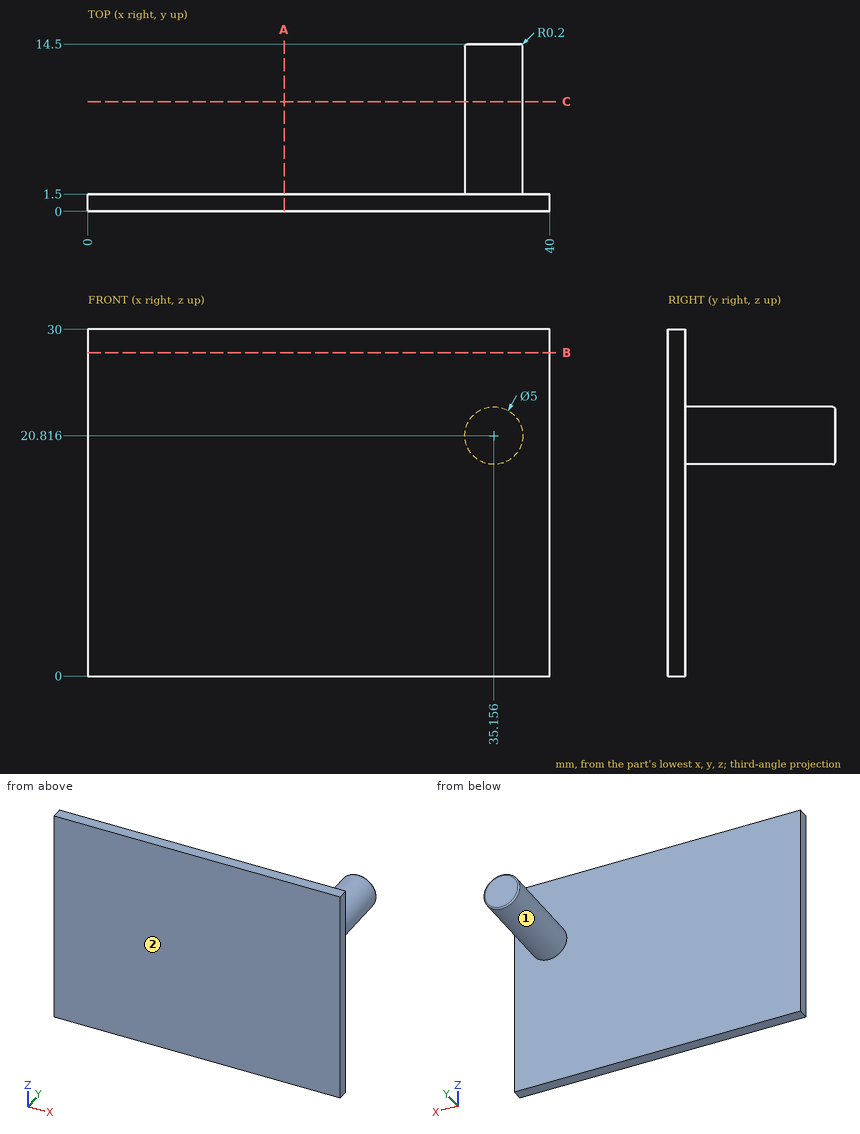
Verification items for this drawing (mm, ordinates from the low corner). A direction names the side the tool comes from. Round coordinates to 2 decimals unless told otherwise and drop trailing zeros. Order: outer loops, then holes, each group sorted by start corner. A loop starts at its lowest first (then second) coordinate and runs counter-clockwise, first axis right, second up.
1) Depth check by flat-ended pin: pin 1 (3 mm diameter, centred on x = 21, z = 16.5, fed in from +Y); pin 2 (12 mm diameter, centred on x = 33.5, z = 3, fed in from -Y); pin 3 (1 mm diameter, centred on y = 9, z = 20, fed in from -X). Enter the tip coordinate at first touch or a pass-through.
Geometry says:
pin 1: stops at y = 1.5
pin 2: stops at y = 0
pin 3: stops at x = 32.68
2) Tool access check on the marked faces 1 and 2. Record the directions out of +Z, -Z, +X, -X, +Y, -Y that give a thin tool (end or side, any length) a straight path to the whole face; none if there is none.
Geometry says:
face 1: +Y
face 2: +Z, -Z, +X, -X, -Y
3) Cross-section at A-A, the plane x = 17. Record the cut outline in (y, z).
Geometry says:
outline: (0, 0) - (1.5, 0) - (1.5, 30) - (0, 30) - close
4) Cross-section at C-C, the plane y = 9.5. Record the cut outline in (x, z) (1 decimal).
Geometry says:
outline: circle Ø5 at (35.2, 20.8)
5) Cross-section at B-B, the plane z = 28. Record the cut outline in (x, y).
Geometry says:
outline: (0, 0) - (40, 0) - (40, 1.5) - (0, 1.5) - close
6) Material ranges on line 1 (Y direction, x = 27, z = 1.5); line 2 (Y direction, x = 35, z = 18.5); line 3 (X direction, y = 5, z = 20), recorded low to high.
Geometry says:
line 1: y = 0 to 1.5
line 2: y = 0 to 14.5
line 3: x = 32.79 to 37.52
